Read the model definition and answer for the solid it produces. Units are mm, in the model's axes. Face numbers are marked on the shaded views. A direction names the side the tool comes from. Round coordinates to 2 decimals unless told otherwise and drop trailing zeros. Loops run counter-clockwise (first coordinate to the right, second up) from the corner with the lowest first, then second, coordinate; pieces in that order, holes last. Notation, with made-up numbers: (-26, -32.5) -> (16, -32.5) arc R25 cw to (16, 0.5) -> close; hole circle Ø3 at (34, 22). An arc over 180 degrees is marked (long way). Put each result on its own line as item: value.
from build123d import *

# Parameters (mm, degrees)
BRIDA_BASE1_DEPTH     = 16
CROQUIS6_R            = 1.5
CORTAR_EXTRUIR6_DEPTH = 0.5
CROQUIS7_R            = 1.5
CORTAR_EXTRUIR7_DEPTH = 0.5
CORTAR_EXTRUIR8_DEPTH = 10


# Sheet-metal steps are written as plain solids
with BuildPart() as part:
    # Croquis1 → Brida base1 (new body)
    with BuildSketch(Plane(origin=(0, 0, 0), x_dir=(1, 0, 0), z_dir=(0, 1, 0))):
        with BuildLine():
            Line((-58.939086294, 3.693519459), (-58.939086294, -15.306480541))
            ThreePointArc((-58.939086294, -15.306480541), (-58.646193076, -16.013587323), (-57.939086294, -16.306480541))
            Line((-57.939086294, -16.306480541), (2.060913706, -16.306480541))
            ThreePointArc((2.060913706, -16.306480541), (2.768020487, -16.013587323), (3.060913706, -15.306480541))
            Line((3.060913706, -15.306480541), (3.060913706, 3.693519459))
            Line((3.060913706, 3.693519459), (2.560913706, 3.693519459))
            Line((2.560913706, 3.693519459), (2.560913706, -15.306480541))
            ThreePointArc((2.560913706, -15.306480541), (2.414467096, -15.660033932), (2.060913706, -15.806480541))
            Line((2.060913706, -15.806480541), (-57.939086294, -15.806480541))
            ThreePointArc((-57.939086294, -15.806480541), (-58.292639685, -15.660033932), (-58.439086294, -15.306480541))
            Line((-58.439086294, -15.306480541), (-58.439086294, 3.693519459))
            Line((-58.439086294, 3.693519459), (-58.939086294, 3.693519459))
        make_face()
    extrude(amount=BRIDA_BASE1_DEPTH)

    # Croquis6 → Cortar-Extruir6 (cut)
    with BuildSketch(Plane(origin=(3.060913706, 0, 0), x_dir=(0, 0, -1), z_dir=(1, 0, 0))):
        with Locations((-11.555105987, 8.25)):
            Circle(CROQUIS6_R)
        with BuildLine():
            Line((-9.595105987, 8.25), (-9.595105987, 0))
            Line((-9.595105987, 0), (3.693519459, 0))
            Line((3.693519459, 0), (3.693519459, 16))
            Line((3.693519459, 16), (-6.095105987, 16))
            Line((-6.095105987, 16), (-6.095105987, 11.75))
            ThreePointArc((-6.095105987, 11.75), (-8.569979721, 10.724873734), (-9.595105987, 8.25))
        make_face()
    extrude(amount=-CORTAR_EXTRUIR6_DEPTH, mode=Mode.SUBTRACT)

    # Croquis7 → Cortar-Extruir7 (cut)
    with BuildSketch(Plane.ZY.offset(58.939086294)):
        with Locations((10.056480541, 8.25)):
            Circle(CROQUIS7_R)
        Polygon((6.095105987, 16), (6.056480541, 0), (-3.693519459, 0), (-3.693519459, 16), align=None)
    extrude(amount=-CORTAR_EXTRUIR7_DEPTH, mode=Mode.SUBTRACT)

    # Croquis8 → Cortar-Extruir8 (cut)
    with BuildSketch(Plane.XY.offset(16.306480541)):
        with BuildLine():
            Line((-50.493414499, 12), (-50.493414499, 3.818786101))
            Line((-50.493414499, 3.818786101), (-50.493414499, 0))
            Line((-50.493414499, 0), (-46.38475809, 0))
            Line((-46.38475809, 0), (-46.38475809, 3.818786101))
            Line((-46.38475809, 3.818786101), (-46.38475809, 12))
            ThreePointArc((-46.38475809, 12), (-48.439086294, 14.054328205), (-50.493414499, 12))
        make_face()
    extrude(amount=-CORTAR_EXTRUIR8_DEPTH, mode=Mode.SUBTRACT)


solid = part.part
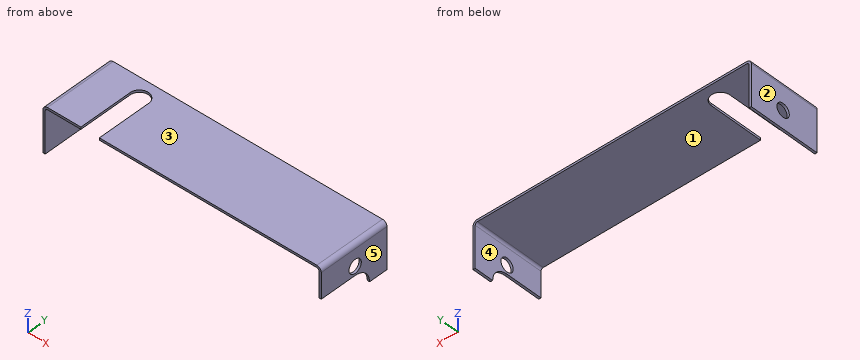
Item 1: Find the intervals of material crossed by line 1 along X through (y, z) = (3.5, 10.75); line 2 along Z through (x, y) = (-5.5, 2.5); line 3 along X through (y, z) = (8.25, 10), in increasing order.
Derived:
line 1: x = -58.94 to -58.44, 2.56 to 3.06
line 2: z = 15.81 to 16.31
line 3: x = 2.56 to 3.06
Item 2: For a pull along X with two mould halves and no side action, classify the marked faces 1, 2 and 3 as pulls with the +X half, pulls with the -X half, needs draft (parallel to the pull), parting line crosses it, or undercut.
Derived:
face 1: undercut
face 2: pulls with the -X half
face 3: needs draft
Item 3: Which of the six approach directions +Z, -Z, +X, -X, +Y, -Y give full straight-line access (tool end or side, diameter ignored) to the marked faces 4 and 5?
Derived:
face 4: -Z, +Y, -Y
face 5: +Z, -Z, +X, +Y, -Y
Item 4: The part is cut by section C-C (y = 7.5). Determine the outline of the cut face in (x, z).
Derived:
outline: (-58.94, 6.07) -> (-58.44, 6.07) -> (-58.44, 8.76) -> (-58.94, 8.76) -> close; (-58.94, 11.36) -> (-58.44, 11.36) -> (-58.44, 15.31) arc R0.5 cw to (-57.94, 15.81) -> (-50.49, 15.81) -> (-50.49, 16.31) -> (-57.94, 16.31) arc R1 ccw to (-58.94, 15.31) -> close; (-46.38, 15.81) -> (2.06, 15.81) arc R0.5 cw to (2.56, 15.31) -> (2.56, 12.85) -> (3.06, 12.85) -> (3.06, 15.31) arc R1 ccw to (2.06, 16.31) -> (-46.38, 16.31) -> close; (2.56, 9.6) -> (3.06, 9.6) -> (3.06, 10.26) -> (2.56, 10.26) -> close
Item 5: The part is cut by section B-B (z = 7.5). Determine the outline of the cut face in (x, y).
Derived:
outline: (-58.94, 0) -> (-58.44, 0) -> (-58.44, 16) -> (-58.94, 16) -> close; (2.56, 11.46) -> (3.06, 11.46) -> (3.06, 16) -> (2.56, 16) -> close
Item 6: The part is cut by section D-D (x = -5.5). Determine the outline of the cut face in (y, z), then the cut area to 3 significant figures.
Derived:
outline: (0, 15.81) -> (16, 15.81) -> (16, 16.31) -> (0, 16.31) -> close
area: 8.00 mm^2
Item 7: Flat-ended cylindrical pins translate along their axes: pin 1 Ø0.6 at (x, y) = (3, 15) entering from -Z; pin 2 Ø0.6 at (x, y) = (3, 2) entering from -Z; pin 3 Ø2.5 at (y, z) = (8.25, 11.56) entering from +X. Find the tip coordinate at first contact, or state that the pin passes through.
Derived:
pin 1: stops at z = 6.1
pin 2: stops at z = 9.6
pin 3: stops at x = -58.44
Item 8: The part is cut by section A-A (y = 12.75). Determine the outline of the cut face in (x, z), then the cut area to 3 significant figures.
Derived:
outline: (-58.94, 6.09) -> (-58.44, 6.09) -> (-58.44, 15.31) arc R0.5 cw to (-57.94, 15.81) -> (-50.35, 15.81) -> (-50.35, 16.31) -> (-57.94, 16.31) arc R1 ccw to (-58.94, 15.31) -> close; (-46.53, 15.81) -> (2.06, 15.81) arc R0.5 cw to (2.56, 15.31) -> (2.56, 6.1) -> (3.06, 6.1) -> (3.06, 15.31) arc R1 ccw to (2.06, 16.31) -> (-46.53, 16.31) -> close
area: 38.5 mm^2
